```python
from build123d import *

# Parameters (mm, degrees)
SKETCH_1_W          = 15
SKETCH_1_H          = 15
SKETCH_1_W_2        = 12
SKETCH_1_H_2        = 12
EXTRUDE_1_DEPTH     = 775
CUT_EXTRUDE_1_REACH = 777.29
SKETCH_2_R          = 2.15
CUT_EXTRUDE_2_REACH = 777.29
SKETCH_3_R          = 2.15


with BuildPart() as part:
    # ｽｹｯﾁ1 → 押し出し-薄板1 (new body)
    with BuildSketch(Plane(origin=(0, 0, 0), x_dir=(1, 0, 0), z_dir=(0, 1, 0))):
        with Locations((7.5, 7.5)):
            Rectangle(SKETCH_1_W, SKETCH_1_H)
        with Locations((7.5, 7.5)):
            Rectangle(SKETCH_1_W_2, SKETCH_1_H_2, mode=Mode.SUBTRACT)
    extrude(amount=EXTRUDE_1_DEPTH)

    # ｶｯﾄ - 押し出し1: up to this face of the body (flat: up to its plane)
    cut_extrude_1_end = Plane(part.part.faces().sort_by_distance((0, 387.5, -7.5))[0])
    # ｽｹｯﾁ2 → ｶｯﾄ - 押し出し1 (cut, up to the picked face)
    with BuildSketch(Plane(origin=(15, 0, 0), x_dir=(0, 0, -1), z_dir=(1, 0, 0)), mode=Mode.PRIVATE) as cut_extrude_1_sk1:
        with Locations((7.5, 10)):
            Circle(SKETCH_2_R)
    cut_extrude_1_tool1 = split(extrude(cut_extrude_1_sk1.sketch, amount=-CUT_EXTRUDE_1_REACH, mode=Mode.PRIVATE), bisect_by=cut_extrude_1_end, keep=Keep.BOTH, mode=Mode.PRIVATE)
    # ｽｹｯﾁ2 → ｶｯﾄ - 押し出し1 (cut, up to the picked face)
    with BuildSketch(Plane(origin=(15, 0, 0), x_dir=(0, 0, -1), z_dir=(1, 0, 0)), mode=Mode.PRIVATE) as cut_extrude_1_sk2:
        with Locations((7.5, 516)):
            Circle(SKETCH_2_R)
    cut_extrude_1_tool2 = split(extrude(cut_extrude_1_sk2.sketch, amount=-CUT_EXTRUDE_1_REACH, mode=Mode.PRIVATE), bisect_by=cut_extrude_1_end, keep=Keep.BOTH, mode=Mode.PRIVATE)
    # ｽｹｯﾁ2 → ｶｯﾄ - 押し出し1 (cut, up to the picked face)
    with BuildSketch(Plane(origin=(15, 0, 0), x_dir=(0, 0, -1), z_dir=(1, 0, 0)), mode=Mode.PRIVATE) as cut_extrude_1_sk3:
        with Locations((7.5, 767.5)):
            Circle(SKETCH_2_R)
    cut_extrude_1_tool3 = split(extrude(cut_extrude_1_sk3.sketch, amount=-CUT_EXTRUDE_1_REACH, mode=Mode.PRIVATE), bisect_by=cut_extrude_1_end, keep=Keep.BOTH, mode=Mode.PRIVATE)
    # ｽｹｯﾁ2 → ｶｯﾄ - 押し出し1 (cut, up to the picked face)
    with BuildSketch(Plane(origin=(15, 0, 0), x_dir=(0, 0, -1), z_dir=(1, 0, 0)), mode=Mode.PRIVATE) as cut_extrude_1_sk4:
        with Locations((7.5, 50)):
            Circle(SKETCH_2_R)
    cut_extrude_1_tool4 = split(extrude(cut_extrude_1_sk4.sketch, amount=-CUT_EXTRUDE_1_REACH, mode=Mode.PRIVATE), bisect_by=cut_extrude_1_end, keep=Keep.BOTH, mode=Mode.PRIVATE)
    # ｽｹｯﾁ2 → ｶｯﾄ - 押し出し1 (cut, up to the picked face)
    with BuildSketch(Plane(origin=(15, 0, 0), x_dir=(0, 0, -1), z_dir=(1, 0, 0)), mode=Mode.PRIVATE) as cut_extrude_1_sk5:
        with Locations((7.5, 536)):
            Circle(SKETCH_2_R)
    cut_extrude_1_tool5 = split(extrude(cut_extrude_1_sk5.sketch, amount=-CUT_EXTRUDE_1_REACH, mode=Mode.PRIVATE), bisect_by=cut_extrude_1_end, keep=Keep.BOTH, mode=Mode.PRIVATE)
    # ｽｹｯﾁ2 → ｶｯﾄ - 押し出し1 (cut, up to the picked face)
    with BuildSketch(Plane(origin=(15, 0, 0), x_dir=(0, 0, -1), z_dir=(1, 0, 0)), mode=Mode.PRIVATE) as cut_extrude_1_sk6:
        with Locations(Location((7.5, 496, 0), (0, 0, 180))):
            Circle(SKETCH_2_R)
    cut_extrude_1_tool6 = split(extrude(cut_extrude_1_sk6.sketch, amount=-CUT_EXTRUDE_1_REACH, mode=Mode.PRIVATE), bisect_by=cut_extrude_1_end, keep=Keep.BOTH, mode=Mode.PRIVATE)
    # ｽｹｯﾁ2 → ｶｯﾄ - 押し出し1 (cut, up to the picked face)
    with BuildSketch(Plane(origin=(15, 0, 0), x_dir=(0, 0, -1), z_dir=(1, 0, 0)), mode=Mode.PRIVATE) as cut_extrude_1_sk7:
        with Locations((7.5, 747.5)):
            Circle(SKETCH_2_R)
    cut_extrude_1_tool7 = split(extrude(cut_extrude_1_sk7.sketch, amount=-CUT_EXTRUDE_1_REACH, mode=Mode.PRIVATE), bisect_by=cut_extrude_1_end, keep=Keep.BOTH, mode=Mode.PRIVATE)
    # ｽｹｯﾁ2 → ｶｯﾄ - 押し出し1 (cut, up to the picked face)
    with BuildSketch(Plane(origin=(15, 0, 0), x_dir=(0, 0, -1), z_dir=(1, 0, 0)), mode=Mode.PRIVATE) as cut_extrude_1_sk8:
        with Locations((7.5, 727.5)):
            Circle(SKETCH_2_R)
    cut_extrude_1_tool8 = split(extrude(cut_extrude_1_sk8.sketch, amount=-CUT_EXTRUDE_1_REACH, mode=Mode.PRIVATE), bisect_by=cut_extrude_1_end, keep=Keep.BOTH, mode=Mode.PRIVATE)
    add(cut_extrude_1_tool1.solids().sort_by(Axis((15, 10, -7.5), (-1, 0, 0)))[0], mode=Mode.SUBTRACT)
    add(cut_extrude_1_tool2.solids().sort_by(Axis((15, 516, -7.5), (-1, 0, 0)))[0], mode=Mode.SUBTRACT)
    add(cut_extrude_1_tool3.solids().sort_by(Axis((15, 767.5, -7.5), (-1, 0, 0)))[0], mode=Mode.SUBTRACT)
    add(cut_extrude_1_tool4.solids().sort_by(Axis((15, 50, -7.5), (-1, 0, 0)))[0], mode=Mode.SUBTRACT)
    add(cut_extrude_1_tool5.solids().sort_by(Axis((15, 536, -7.5), (-1, 0, 0)))[0], mode=Mode.SUBTRACT)
    add(cut_extrude_1_tool6.solids().sort_by(Axis((15, 496, -7.5), (-1, 0, 0)))[0], mode=Mode.SUBTRACT)
    add(cut_extrude_1_tool7.solids().sort_by(Axis((15, 747.5, -7.5), (-1, 0, 0)))[0], mode=Mode.SUBTRACT)
    add(cut_extrude_1_tool8.solids().sort_by(Axis((15, 727.5, -7.5), (-1, 0, 0)))[0], mode=Mode.SUBTRACT)

    # ｶｯﾄ - 押し出し2: up to this face of the body (flat: up to its plane)
    cut_extrude_2_end = Plane(part.part.faces().sort_by_distance((7.5, 387.5, -15))[0])
    # ｽｹｯﾁ3 → ｶｯﾄ - 押し出し2 (cut, up to the picked face)
    with BuildSketch(Plane.XY, mode=Mode.PRIVATE) as cut_extrude_2_sk1:
        with Locations((7.5, 685)):
            Circle(SKETCH_3_R)
    cut_extrude_2_tool1 = split(extrude(cut_extrude_2_sk1.sketch, amount=-CUT_EXTRUDE_2_REACH, mode=Mode.PRIVATE), bisect_by=cut_extrude_2_end, keep=Keep.BOTH, mode=Mode.PRIVATE)
    # ｽｹｯﾁ3 → ｶｯﾄ - 押し出し2 (cut, up to the picked face)
    with BuildSketch(Plane.XY, mode=Mode.PRIVATE) as cut_extrude_2_sk2:
        with Locations((7.5, 655)):
            Circle(SKETCH_3_R)
    cut_extrude_2_tool2 = split(extrude(cut_extrude_2_sk2.sketch, amount=-CUT_EXTRUDE_2_REACH, mode=Mode.PRIVATE), bisect_by=cut_extrude_2_end, keep=Keep.BOTH, mode=Mode.PRIVATE)
    # ｽｹｯﾁ3 → ｶｯﾄ - 押し出し2 (cut, up to the picked face)
    with BuildSketch(Plane.XY, mode=Mode.PRIVATE) as cut_extrude_2_sk3:
        with Locations((7.5, 605)):
            Circle(SKETCH_3_R)
    cut_extrude_2_tool3 = split(extrude(cut_extrude_2_sk3.sketch, amount=-CUT_EXTRUDE_2_REACH, mode=Mode.PRIVATE), bisect_by=cut_extrude_2_end, keep=Keep.BOTH, mode=Mode.PRIVATE)
    # ｽｹｯﾁ3 → ｶｯﾄ - 押し出し2 (cut, up to the picked face)
    with BuildSketch(Plane.XY, mode=Mode.PRIVATE) as cut_extrude_2_sk4:
        with Locations((7.5, 575)):
            Circle(SKETCH_3_R)
    cut_extrude_2_tool4 = split(extrude(cut_extrude_2_sk4.sketch, amount=-CUT_EXTRUDE_2_REACH, mode=Mode.PRIVATE), bisect_by=cut_extrude_2_end, keep=Keep.BOTH, mode=Mode.PRIVATE)
    # ｽｹｯﾁ3 → ｶｯﾄ - 押し出し2 (cut, up to the picked face)
    with BuildSketch(Plane.XY, mode=Mode.PRIVATE) as cut_extrude_2_sk5:
        with Locations((7.5, 27.5)):
            Circle(SKETCH_3_R)
    cut_extrude_2_tool5 = split(extrude(cut_extrude_2_sk5.sketch, amount=-CUT_EXTRUDE_2_REACH, mode=Mode.PRIVATE), bisect_by=cut_extrude_2_end, keep=Keep.BOTH, mode=Mode.PRIVATE)
    add(cut_extrude_2_tool1.solids().sort_by(Axis((7.5, 685, 0), (0, 0, -1)))[0], mode=Mode.SUBTRACT)
    add(cut_extrude_2_tool2.solids().sort_by(Axis((7.5, 655, 0), (0, 0, -1)))[0], mode=Mode.SUBTRACT)
    add(cut_extrude_2_tool3.solids().sort_by(Axis((7.5, 605, 0), (0, 0, -1)))[0], mode=Mode.SUBTRACT)
    add(cut_extrude_2_tool4.solids().sort_by(Axis((7.5, 575, 0), (0, 0, -1)))[0], mode=Mode.SUBTRACT)
    add(cut_extrude_2_tool5.solids().sort_by(Axis((7.5, 27.5, 0), (0, 0, -1)))[0], mode=Mode.SUBTRACT)


solid = part.part
```
Work out the finished part from the listing and answer in its coordinate system (mm). A direction names the side the tool comes from. Give positions to 0.01 mm unless a question says otherwise; leave off trailing zeros. Order: outer loops, then holes, each group sorted by start corner. A loop starts at its lowest first (then second) coordinate and runs counter-clockwise, first axis right, second up. Notation, with made-up numbers: M 38.25,-29.5 L 52.25,-29.5 A14 ccw 52.25,-12.5 Z; hole C -7,51.5 d3. An arc over 180 degrees is marked long. Return JSON: item names as keys, results as strings.
1) This flat-tipped pin is pushed along its axis until it touches: pin 1 (3.5 mm diameter, centred on x = 7.5, y = 655, fed in from -Z). Where does it stop, or does it pass through?
Resolved:
{"pin 1": "through"}
2) A tool of negligible diameter and unlimited length cuts with its end or side. For faces 1 (the flat face through (7, 382, -1.5)), 2 (the flat face through (14, 0, -8)), from which of +Z, -Z, +X, -X, +Y, -Y can it reach the whole face along a straight path? Write none if from no direction.
Resolved:
{"face 1": "+Y, -Y", "face 2": "+Z, -Z, +X, -X, -Y"}
3) Section A-A, the plane y = 293.5 is taken. Write down the section's boundary in (x, z).
Resolved:
{"outline": "M 0,-15 L 15,-15 L 15,0 L 0,0 Z; hole M 1.5,-13.5 L 13.5,-13.5 L 13.5,-1.5 L 1.5,-1.5 Z"}
4) Straight lines are drawn through the part: line 1 along Z through (x, y) = (11.25, 629); line 2 along Z through (x, y) = (0.9, 496); line 3 along X through (y, z) = (346.5, -3.5). For each, find the intervals that lie inside material, in ascending order. Write a range as [from, to].
Resolved:
{"line 1": "[-15, -13.5], [-1.5, 0]", "line 2": "[-15, -9.65], [-5.35, 0]", "line 3": "[0, 1.5], [13.5, 15]"}
5) For a pull along Z with two mould halves and no side action, classify faces 3 (the flat face through (7, 382, 0)), 4 (the flat face through (1.5, 382, -7)), 5 (the flat face through (7, 382, -15)), 6 (the flat face through (0, 382, -7)) as +Z half, -Z half, draft (parallel to the pull), parting line (faces both ways), or undercut.
Resolved:
{"face 3": "+Z half", "face 4": "undercut", "face 5": "-Z half", "face 6": "draft"}
